from build123d import *

# Parameters (mm, degrees)
SKETCH1_R               = 68
SKETCH1_R_2             = 56
SKETCH1_R_3             = 1.6
BOSS_EXTRUDE1_DEPTH     = 20
SKETCH2_R               = 76
CUT_EXTRUDE1_DEPTH      = 99.224233262
CUT_EXTRUDE2_REACH      = 163.628
CUT_EXTRUDE2_END_RADIUS = 56
SKETCH3_R               = 1.6
CIRPATTERN4_COUNT       = 8
FILLET1_R               = 10


with BuildPart() as part:
    # Sketch1 → Boss-Extrude1 (new body)
    with BuildSketch(Plane(origin=(0, 0, 0), x_dir=(1, 0, 0), z_dir=(0, 1, 0))):
        with Locations(Location((0, 0, 0), (0, 0, 270))):
            Circle(SKETCH1_R)
        with Locations(Location((0, 0, 0), (0, 0, 270))):
            Circle(SKETCH1_R_2, mode=Mode.SUBTRACT)
        with Locations(Location((0, 62, 0), (0, 0, 270))):
            Circle(SKETCH1_R_3, mode=Mode.SUBTRACT)
        with Locations(Location((43.840620434, 43.840620434, 0), (0, 0, 270))):
            Circle(SKETCH1_R_3, mode=Mode.SUBTRACT)
        with Locations(Location((62, 0, 0), (0, 0, 270))):
            Circle(SKETCH1_R_3, mode=Mode.SUBTRACT)
        with Locations(Location((43.840620434, -43.840620434, 0), (0, 0, 270))):
            Circle(SKETCH1_R_3, mode=Mode.SUBTRACT)
        with Locations(Location((0, -62, 0), (0, 0, 270))):
            Circle(SKETCH1_R_3, mode=Mode.SUBTRACT)
        with Locations(Location((-43.840620434, -43.840620434, 0), (0, 0, 270))):
            Circle(SKETCH1_R_3, mode=Mode.SUBTRACT)
        with Locations(Location((-62, 0, 0), (0, 0, 270))):
            Circle(SKETCH1_R_3, mode=Mode.SUBTRACT)
        with Locations(Location((-43.840620434, 43.840620434, 0), (0, 0, 270))):
            Circle(SKETCH1_R_3, mode=Mode.SUBTRACT)
    extrude(amount=BOSS_EXTRUDE1_DEPTH)

    # Sketch2 → Cut-Extrude1 (cut, through all)
    with BuildSketch(Plane(origin=(0, 20, 0), x_dir=(1, 0, 0), z_dir=(0, 1, 0))):
        Circle(SKETCH2_R)
        with BuildLine():
            Line((16.500755195, 65.967606278), (34.978345845, 58.31393763))
            ThreePointArc((34.978345845, 58.31393763), (48.083261121, 48.083261121), (58.31393763, 34.978345845))
            Line((58.31393763, 34.978345845), (65.967606278, 16.500755195))
            ThreePointArc((65.967606278, 16.500755195), (68, 0), (65.967606278, -16.500755195))
            Line((65.967606278, -16.500755195), (58.31393763, -34.978345845))
            ThreePointArc((58.31393763, -34.978345845), (48.083261121, -48.083261121), (34.978345845, -58.31393763))
            Line((34.978345845, -58.31393763), (16.500755195, -65.967606278))
            ThreePointArc((16.500755195, -65.967606278), (0, -68), (-16.500755195, -65.967606278))
            Line((-16.500755195, -65.967606278), (-34.978345845, -58.31393763))
            ThreePointArc((-34.978345845, -58.31393763), (-48.083261121, -48.083261121), (-58.31393763, -34.978345845))
            Line((-58.31393763, -34.978345845), (-65.967606278, -16.500755195))
            ThreePointArc((-65.967606278, -16.500755195), (-68, 0), (-65.967606278, 16.500755195))
            Line((-65.967606278, 16.500755195), (-58.31393763, 34.978345845))
            ThreePointArc((-58.31393763, 34.978345845), (-48.083261121, 48.083261121), (-34.978345845, 58.31393763))
            Line((-34.978345845, 58.31393763), (-16.500755195, 65.967606278))
            ThreePointArc((-16.500755195, 65.967606278), (0, 68), (16.500755195, 65.967606278))
        make_face(mode=Mode.SUBTRACT)
    extrude(amount=-CUT_EXTRUDE1_DEPTH, mode=Mode.SUBTRACT)

    # Cut-Extrude2: up to this cylinder (the profile starts outside it)
    cut_extrude2_end = Plane(origin=(0, 10, 0), z_dir=(0, -1, 0)) * Cylinder(CUT_EXTRUDE2_END_RADIUS, 440.256, mode=Mode.PRIVATE)
    # Sketch3 → Cut-Extrude2 (cut, up to the surface)
    with BuildSketch(Plane(origin=(-25.73955052, 0, -62.140771954), x_dir=(-0.9238795325112866, 0, 0.38268343236509017), z_dir=(-0.3826834323650902, 0, -0.9238795325112867)), mode=Mode.PRIVATE) as cut_extrude2_sk1:
        with Locations((0, 10)):
            Circle(SKETCH3_R)
    cut_extrude2_tool1 = extrude(cut_extrude2_sk1.sketch, amount=-CUT_EXTRUDE2_REACH, mode=Mode.PRIVATE) - cut_extrude2_end
    cut_extrude2 = cut_extrude2_tool1.solids().sort_by_distance((-25.739551, 10, -62.140772))[0]
    add(cut_extrude2, mode=Mode.SUBTRACT)

    # CirPattern4: Cut-Extrude2 ×8 about axis
    cirpattern4_axis = Axis((0, 20, 0), (0, 1, 0))
    for i in range(1, CIRPATTERN4_COUNT):
        add(cut_extrude2.rotate(cirpattern4_axis, i * 360 / CIRPATTERN4_COUNT), mode=Mode.SUBTRACT)

    # Fillet1
    fillet1_edges = [part.edges().sort_by_distance(p)[0] for p in [
        (16.500755195, 10, -65.967606278),
        (34.978345845, 10, -58.31393763),
        (58.31393763, 10, -34.978345845),
        (65.967606278, 10, -16.500755195),
        (65.967606278, 10, 16.500755195),
        (58.31393763, 10, 34.978345845),
        (34.978345845, 10, 58.31393763),
        (16.500755195, 10, 65.967606278),
        (-16.500755195, 10, 65.967606278),
        (-34.978345845, 10, 58.31393763),
        (-58.31393763, 10, 34.978345845),
        (-65.967606278, 10, 16.500755195),
        (-65.967606278, 10, -16.500755195),
        (-58.31393763, 10, -34.978345845),
        (-34.978345845, 10, -58.31393763),
        (-16.500755195, 10, -65.967606278),
    ]]
    fillet(fillet1_edges, radius=FILLET1_R)


solid = part.part
Model file for the job. Use its own axes, mm. Coordinates: 2 decimals unless noted, no trailing zeros. Order: outer loops, then holes, each group sorted by start corner. A loop starts at its lowest first (then second) coordinate and runs counter-clockwise, first axis right, second up. Notation, with made-up numbers: M -13.75,-38.5 L 19.25,-38.5 A21 cw 19.25,-27.5 Z; hole C -22.75,62 d8. An arc over 180 degrees is marked long. Return JSON: item names as keys, results as strings.
1. Saw through at D-D (y = 18). Give the number of separate pieces and of enclosed holes in the cut face, and give its area (3 significant figures).
Ans:
{"separate pieces": "1", "enclosed holes": "9", "area": "4,530 mm^2"}
2. Pull direction Y, two halves, no side cores. Call faces 1 (the face through (-23.725, 10.14, 62.975)), 2 (the face through (-50, 0, -26)), 3 (the face through (-57.134, 8.438, 23.29)): +Y half, -Y half, draft (parallel to the pull), parting line (faces both ways), or undercut.
Ans:
{"face 1": "draft", "face 2": "-Y half", "face 3": "undercut"}
3. Flat gauge pins, fed straight in: pin 1 (1.5 mm diameter, centred on x = 30, y = 12, fed in from +Z); pin 2 (3 mm diameter, centred on x = 0, z = -62, fed in from +Y); pin 3 (1 mm diameter, centred on x = 4, y = 14, fed in from -Z); pin 4 (10 mm diameter, centred on x = -13, y = 2.5, fed in from -Z). Where does each tip first touch, or does it go through?
Ans:
{"pin 1": "z = 60.69", "pin 2": "through", "pin 3": "z = -67.91", "pin 4": "z = -67.53"}
4. Saw through at A-A (z = 0). Give the cut face in (x, y), and give its area (3 significant figures).
Ans:
{"outline": "M -68,0 L -63.6,0 L -63.6,20 L -68,20 Z; M -60.4,0 L -56,0 L -56,20 L -60.4,20 Z; M 56,0 L 60.4,0 L 60.4,20 L 56,20 Z; M 63.6,0 L 68,0 L 68,20 L 63.6,20 Z", "area": "352 mm^2"}
5. Saw through at B-B (x = 0). Give the cut face in (y, z).
Ans:
{"outline": "M 0,-68 L 20,-68 L 20,-63.6 L 0,-63.6 Z; M 0,-60.4 L 20,-60.4 L 20,-56 L 0,-56 Z; M 0,56 L 20,56 L 20,60.4 L 0,60.4 Z; M 0,63.6 L 20,63.6 L 20,68 L 0,68 Z"}
6. Saw through at C-C (z = 47). Give the cut face in (x, y), and give its area (3 significant figures).
Ans:
{"outline": "M -49.14,0 L -30.45,0 L -30.45,20 L -49.14,20 Z; M 30.45,0 L 49.14,0 L 49.14,20 L 30.45,20 Z", "area": "748 mm^2"}
7. Drill centre lines: probe 1 along X at (y, z) = (10, 0); probe 2 along Z at (x, y) = (-57.5, 9.25); probe 3 along Z at (x, y) = (-1, 1.75). Where is each one in solid material? Low to high.
Ans:
{"probe 1": "-68 to -63.6, -60.4 to -56, 56 to 60.4, 63.6 to 68", "probe 2": "-36.3 to -25.35, -22.29 to 22.29, 25.35 to 36.3", "probe 3": "-67.99 to -63.25, -60.75 to -55.99, 55.99 to 60.75, 63.25 to 67.99"}
